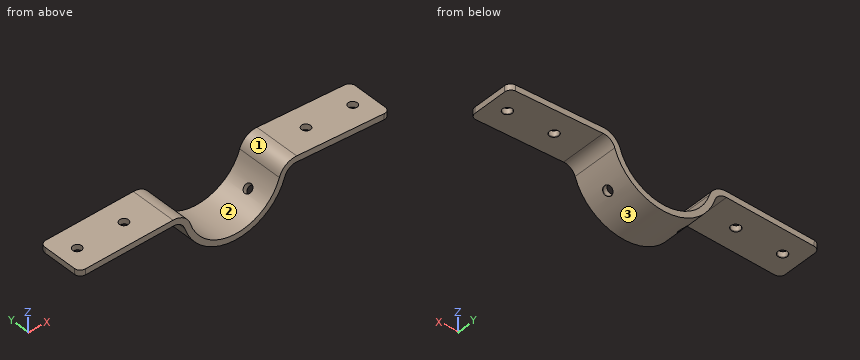
from build123d import *

# Parameters (mm, degrees)
BASE_FLANGE1_DEPTH                    = 12.7
F_11_0_191_DIAMETER_HOLE2_AT_2_COUNT  = 2
F_11_0_191_DIAMETER_HOLE2_AT_2_PITCH  = 25.4
F_11_0_191_DIAMETER_HOLE3_D           = 4.8514
F_11_0_191_DIAMETER_HOLE3_DEPTH       = 40.176204246
F_11_0_191_DIAMETER_HOLE3_CSINK_D     = 5.1562
F_11_0_191_DIAMETER_HOLE3_CSINK_ANGLE = 45
FILLET2_R                             = 3.175


# Sheet-metal steps are written as plain solids
with BuildPart() as part:
    # Sketch1 → Base-Flange1 (new, symmetric)
    with BuildSketch(Plane(origin=(0, 0, 0), x_dir=(1, 0, 0), z_dir=(0, 1, 0))):
        with BuildLine():
            Line((84.349626816, 2.945553875), (33.580572804, 1.172659442))
            ThreePointArc((33.580572804, 1.172659442), (27.77304054, 2.897708907), (24.180476435, 7.775896051))
            ThreePointArc((24.180476435, 7.775896051), (0, 25.4), (-24.180476435, 7.775896051))
            ThreePointArc((-24.180476435, 7.775896051), (-27.77304054, 2.897708907), (-33.580572804, 1.172659442))
            Line((-33.580572804, 1.172659442), (-84.349626816, 2.945553875))
            Line((-84.349626816, 2.945553875), (-84.238820914, 6.118619751))
            Line((-84.238820914, 6.118619751), (-33.469766902, 4.345725318))
            ThreePointArc((-33.469766902, 4.345725318), (-29.598078726, 5.495758295), (-27.203035989, 8.747883057))
            ThreePointArc((-27.203035989, 8.747883057), (0, 28.575), (27.203035989, 8.747883057))
            ThreePointArc((27.203035989, 8.747883057), (29.598078726, 5.495758295), (33.469766902, 4.345725318))
            Line((33.469766902, 4.345725318), (84.238820914, 6.118619751))
            Line((84.238820914, 6.118619751), (84.349626816, 2.945553875))
        make_face()
    extrude(amount=BASE_FLANGE1_DEPTH, both=True)

    # Sketch8 → #11 (0.191) Diameter Hole2 (revolve, cut)
    with BuildSketch(Plane(origin=(74.719623287, 0, -5.786202044), x_dir=(-0.9993908270190958, 0, 0.03489949670250169), z_dir=(0, 1, 0))):
        Polygon((0, 0), (0, 4.947848723), (2.4257, 4.947848723), (2.4257, 0.367926147), (2.5781, 0), align=None)
    f_11_0_191_diameter_hole2 = revolve(axis=Axis((74.498011483, 0, -12.132333796), (0.03489949670250171, 0, 0.9993908270190958)), mode=Mode.SUBTRACT)

    # #11 (0.191) Diameter Hole2 at 2: #11 (0.191) Diameter Hole2 ×2
    with Locations(*[Vector(-0.9993908270190958, 0, 0.034899496702501684) * (i * F_11_0_191_DIAMETER_HOLE2_AT_2_PITCH) for i in range(1, F_11_0_191_DIAMETER_HOLE2_AT_2_COUNT)]):
        add(f_11_0_191_diameter_hole2, mode=Mode.SUBTRACT)

    # #11 (0.191) Diameter Hole3
    with Locations(Plane(origin=(20.205576272, 0, -20.205576272), x_dir=(0.707106781187, 0, 0.707106781187), z_dir=(0.707106781187, 0, -0.707106781187))):
        with Locations((0, 0)):
            f_11_0_191_diameter_hole3 = CounterSinkHole(F_11_0_191_DIAMETER_HOLE3_D / 2, F_11_0_191_DIAMETER_HOLE3_CSINK_D / 2, depth=F_11_0_191_DIAMETER_HOLE3_DEPTH, counter_sink_angle=F_11_0_191_DIAMETER_HOLE3_CSINK_ANGLE)

    # Fillet2
    fillet2_edges = [part.edges().sort_by_distance(p)[0] for p in [
        (84.294223865, 12.7, -4.532086813),
        (-84.294223865, -12.7, -4.532086813),
        (84.294223865, -12.7, -4.532086813),
        (-84.294223865, 12.7, -4.532086813),
    ]]
    fillet(fillet2_edges, radius=FILLET2_R)

    # Mirror1: #11 (0.191) Diameter Hole2, #11 (0.191) Diameter Hole3 across plane
    add(f_11_0_191_diameter_hole2.mirror(Plane(origin=(0, 0, 0), x_dir=(0, 0, 1), z_dir=(1, 0, 0))), mode=Mode.SUBTRACT)
    add(f_11_0_191_diameter_hole3.mirror(Plane(origin=(0, 0, 0), x_dir=(0, 0, 1), z_dir=(1, 0, 0))), mode=Mode.SUBTRACT)

    # Mirror1 copy 1 sketch → Mirror1 copy 1 (revolve, cut)
    with BuildSketch(Plane(origin=(-49.335096281, 0, -4.899754828), x_dir=(0.9993908270190958, 0, 0.03489949670250169), z_dir=(0, 1, 0))):
        Polygon((0, 0), (0, -4.947848723), (2.4257, -4.947848723), (2.4257, -0.367926147), (2.5781, 0), align=None)
    revolve(axis=Axis((-49.113484477, 0, -11.24588658), (0.03489949670250171, 0, -0.9993908270190958)), mode=Mode.SUBTRACT)


solid = part.part
CAD build for the part. Positions are in the model's coordinates, mm. Face numbers are marked on the shaded views. Coordinates: 2 decimals unless noted, no trailing zeros. Loops run counter-clockwise (first coordinate to the right, second up) from the corner with the lowest first, then second, coordinate; pieces in that order, holes last. Notation, with made-up numbers: (38, -38) - (51, -38) arc R16 cw to (51, -28) - close; hole circle Ø10 at (-21.5, -37.5). An arc over 180 degrees is marked (long way). Write item = value, one per line. Start each with the question number.
Q1. Flat gauge pins, fed straight in: pin 1 Ø2 at (y, z) = (4, -24.5) entering from -X; pin 2 Ø5 at (y, z) = (4, -15) entering from -X; pin 3 Ø1 at (y, z) = (4, -8) entering from -X. Where does each tip first touch, or does it go through?
Q2. Cut at B-B, the plane z = -23.5. List the corners of the cut face in (x, y), then the cut area to 3 significant figures.
Q3. Cut at A-A, the plane y = -5. List the corners of the cut face in (x, z) (3 decimals).
Q4. Pull direction X, two halves, no side cores. Call the marked faces 1, 2 and 3: pulls with the +X half, pulls with the -X half, needs draft (parallel to the pull), parting line crosses it, or undercut.
Q5. Drill centre lines: L1, parallel to X at y = 7.75, z = -14.5; L2, parallel to X at y = 7.75, z = -7.25; L3, parallel to Z at x = -59, y = 7. Where is each one in solid material? Low to high.
Q6. Cut at C-C, the plane x = 1.5. List the corners of the cut face in (y, z).
Q7. Cut at D-D, the plane x = 67.5. List the corners of the cut face in (y, z), then the cut area to 3 significant figures.
Computed:
q1.pin_1 = -16.26
q1.pin_2 = -25.7
q1.pin_3 = -27.76
q2.outline = (-16.26, -12.7) - (-9.64, -12.7) - (-9.64, 12.7) - (-16.26, 12.7) - close; (9.64, -12.7) - (16.26, -12.7) - (16.26, 12.7) - (9.64, 12.7) - close
q2.area = 336 mm²
q3.outline = (-84.35, -2.946) - (-84.239, -6.119) - (-33.47, -4.346) arc R6.35 cw to (-27.203, -8.748) arc R28.575 ccw to (27.203, -8.748) arc R6.35 cw to (33.47, -4.346) - (84.239, -6.119) - (84.35, -2.946) - (33.581, -1.173) arc R9.525 ccw to (24.18, -7.776) arc R25.4 cw to (-24.18, -7.776) arc R9.525 ccw to (-33.581, -1.173) - close
q4.face_1 = undercut
q4.face_2 = undercut
q4.face_3 = parting line crosses it
q5.L1 = -24.62 to -20.85, 20.85 to 24.62
q5.L2 = -27.91 to -24.37, 24.37 to 27.91
q5.L3 = -5.24 to -2.06
q6.outline = (-12.7, -28.54) - (12.7, -28.54) - (12.7, -25.36) - (-12.7, -25.36) - close
q7.outline = (-12.7, -5.53) - (12.7, -5.53) - (12.7, -2.36) - (-12.7, -2.36) - close
q7.area = 80.7 mm²
